Job drawing, mm, ordinate dimensions from the low corner. One solid piece. Give positions to 0.01 mm unless a question says otherwise; leave off trailing zeros. Loops run counter-clockwise (first coordinate to the right, second up) from the corner with the lowest first, then second, coordinate; pieces in that order, holes last. Notation, with made-up numbers: (-11.75, 54.5) -> (-5.75, 54.5) arc R20 cw to (-5.75, 92.5) -> close; hole circle Ø2 at (66, -19). An arc over 180 degrees is marked (long way). Answer as a JSON object with one key per item and string values. Group by question number.
Q1. Band-saw the part on B-B, the plane y = 3.75. Write the cut outline in (x, z), plus the area to 3 significant figures.
Q2. Drop a flat-ended pin along its axis: pin 1 (2 mm diameter, centred on x = 4, y = 3.5, fed in from -Z). Give the stop position or say it passes through.
Q3. Band-saw the part on C-C, the plane x = 11.75. Write the cut outline in (y, z).
Q4. Wall check: probe 1 along Z at (x, y) = (6.35, 3.5); probe 2 along Z at (x, y) = (8.25, 3); probe 3 along Z at (x, y) = (10.75, 0.5). Give the ranges that are in metal, low to high. Write a range as from..to.
Q5. Band-saw the part on A-A, the plane x = 6.35. Write the cut outline in (y, z).
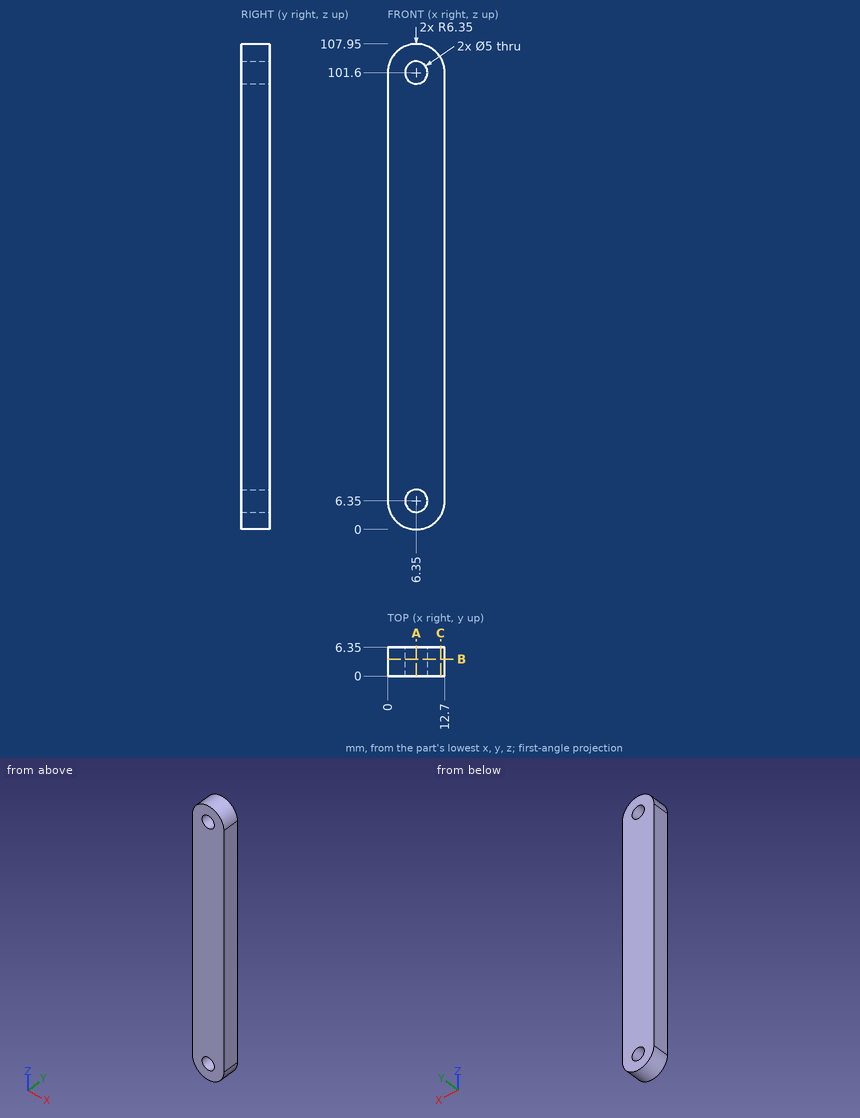
Worked answers:
{
 "1": {"outline": "(0, 6.35) arc R6.35 ccw to (12.7, 6.35) -> (12.7, 101.6) arc R6.35 ccw to (0, 101.6) -> close; hole circle Ø5 at (6.35, 6.35); hole circle Ø5 at (6.35, 101.6)", "area": "1,300 mm2"},
 "2": {"pin 1": "z = 0.15"},
 "3": {"outline": "(0, 3.01) -> (6.35, 3.01) -> (6.35, 104.94) -> (0, 104.94) -> close"},
 "4": {"probe 1": "0..3.85, 8.85..99.1, 104.1..107.95", "probe 2": "0.29..4.73, 7.97..99.98, 103.22..107.66", "probe 3": "1.77..106.18"},
 "5": {"outline": "(0, 0) -> (6.35, 0) -> (6.35, 3.85) -> (0, 3.85) -> close; (0, 8.85) -> (6.35, 8.85) -> (6.35, 99.1) -> (0, 99.1) -> close; (0, 104.1) -> (6.35, 104.1) -> (6.35, 107.95) -> (0, 107.95) -> close"}
}
